Geometry: final body of the model. Coordinates: model frame, mm. Face numbers are marked on the shaded views. A direction names the side the tool comes from. Give positions to 0.01 mm unless a question says otherwise; leave off trailing zeros. Loops run counter-clockwise (first coordinate to the right, second up) from the corner with the lowest first, then second, coordinate; pieces in that order, holes last. Notation, with made-up numbers: M 58,41 L 105,41 A32 cw 105,80 Z; hole C -8.75,-22.5 d8. An arc over 180 degrees is marked long. Put each result on its own line as item: value.
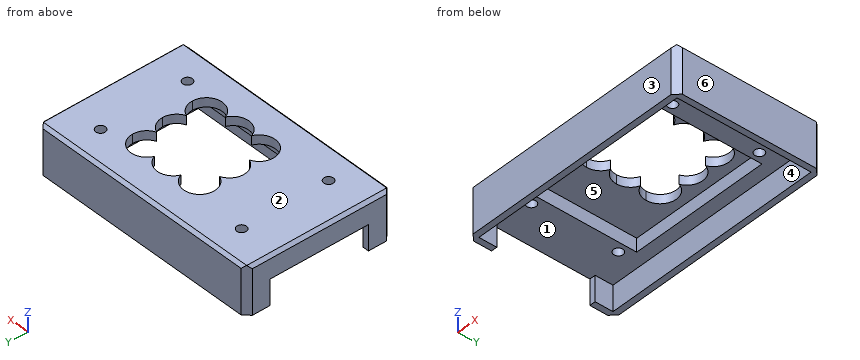
```python
from build123d import *

# Parameters (mm, degrees)
BOSS_EXTRUDE1_START      = 4.485
SKETCH1_W                = 75
SKETCH1_H                = 45
SKETCH1_R                = 1.6
SKETCH1_W_2              = 47.4
SKETCH1_H_2              = 36.3
BOSS_EXTRUDE1_DEPTH      = 3
SKETCH1_4_W              = 75
SKETCH1_4_H              = 45
SKETCH1_4_R              = 1.6
SKETCH1_4_W_2            = 47.4
SKETCH1_4_H_2            = 36.3
BOSS_EXTRUDE2_DEPTH      = 4.485
BOSS_EXTRUDE3_DEPTH      = 8.5
BOSS_EXTRUDE3_DEPTH_BACK = 7.485
SKETCH2_W                = 79
SKETCH2_H                = 49
SKETCH2_W_2              = 75
SKETCH2_H_2              = 45
SKETCH4_W                = 8.5
SKETCH4_H                = 33
CUT_EXTRUDE1_DEPTH       = 52
CHAMFER1_SIZE            = 1
CHAMFER2_SIZE            = 2


with BuildPart() as part:
    # Sketch1 → Boss-Extrude1 (new body)
    # profile 1 of 2: a face of its own
    with BuildSketch(Plane.XY.offset(BOSS_EXTRUDE1_START)):
        with Locations((-52, -40.55)):
            Rectangle(SKETCH1_W, SKETCH1_H)
        with Locations(Location((-78.6, -55.1, 0), (0, 0, 270))):
            Circle(SKETCH1_R, mode=Mode.SUBTRACT)
        with Locations(Location((-78.6, -25.9, 0), (0, 0, 270))):
            Circle(SKETCH1_R, mode=Mode.SUBTRACT)
        with Locations(Location((-25.2, -25.9, 0), (0, 0, 270))):
            Circle(SKETCH1_R, mode=Mode.SUBTRACT)
        with Locations(Location((-25.2, -55.1, 0), (0, 0, 270))):
            Circle(SKETCH1_R, mode=Mode.SUBTRACT)
        with Locations((-51.9, -40.55)):
            Rectangle(SKETCH1_W_2, SKETCH1_H_2, mode=Mode.SUBTRACT)
    # profile 2 of 2: a face of its own
    with BuildSketch(Plane.XY.offset(BOSS_EXTRUDE1_START)):
        with Locations((-51.9, -40.55)):
            Rectangle(SKETCH1_W_2, SKETCH1_H_2)
        with BuildLine():
            ThreePointArc((-35.396713369, -35.7), (-32.895168364, -33.736438417), (-31.95, -30.7))
            ThreePointArc((-31.95, -30.7), (-36.332399876, -25.438227485), (-42.3, -28.796713369))
            ThreePointArc((-42.3, -28.796713369), (-47.3, -25.35), (-52.3, -28.796713369))
            ThreePointArc((-52.3, -28.796713369), (-58.267600124, -25.438227485), (-62.65, -30.7))
            ThreePointArc((-62.65, -30.7), (-61.704831636, -33.736438417), (-59.203286631, -35.7))
            ThreePointArc((-59.203286631, -35.7), (-61.704831636, -37.663561583), (-62.65, -40.7))
            ThreePointArc((-62.65, -40.7), (-61.704831636, -43.736438417), (-59.203286631, -45.7))
            ThreePointArc((-59.203286631, -45.7), (-61.704831636, -47.663561583), (-62.65, -50.7))
            ThreePointArc((-62.65, -50.7), (-58.267600124, -55.961772515), (-52.3, -52.603286631))
            ThreePointArc((-52.3, -52.603286631), (-47.3, -56.05), (-42.3, -52.603286631))
            ThreePointArc((-42.3, -52.603286631), (-36.332399876, -55.961772515), (-31.95, -50.7))
            ThreePointArc((-31.95, -50.7), (-32.895168364, -47.663561583), (-35.396713369, -45.7))
            ThreePointArc((-35.396713369, -45.7), (-32.895168364, -43.736438417), (-31.95, -40.7))
            ThreePointArc((-31.95, -40.7), (-32.895168364, -37.663561583), (-35.396713369, -35.7))
        make_face(mode=Mode.SUBTRACT)
    extrude(amount=BOSS_EXTRUDE1_DEPTH)

    # Sketch1<4> → Boss-Extrude2 (add)
    with BuildSketch(Plane.XY):
        with Locations((-52, -40.55)):
            Rectangle(SKETCH1_4_W, SKETCH1_4_H)
        with Locations((-78.6, -55.1)):
            Circle(SKETCH1_4_R, mode=Mode.SUBTRACT)
        with Locations((-78.6, -25.9)):
            Circle(SKETCH1_4_R, mode=Mode.SUBTRACT)
        with Locations((-25.2, -25.9)):
            Circle(SKETCH1_4_R, mode=Mode.SUBTRACT)
        with Locations((-25.2, -55.1)):
            Circle(SKETCH1_4_R, mode=Mode.SUBTRACT)
        with Locations((-51.9, -40.55)):
            Rectangle(SKETCH1_4_W_2, SKETCH1_4_H_2, mode=Mode.SUBTRACT)
    extrude(amount=BOSS_EXTRUDE2_DEPTH)

    # Sketch2 → Boss-Extrude3 (add, two sides: drawn at the far end of the back side and taken through both)
    with BuildSketch(Plane(origin=(0, 0, 0), x_dir=(-1, 0, 0), z_dir=(0, 0, -1)).offset(-BOSS_EXTRUDE3_DEPTH_BACK)):
        with Locations((52, -40.55)):
            Rectangle(SKETCH2_W, SKETCH2_H)
        with Locations((52, -40.55)):
            Rectangle(SKETCH2_W_2, SKETCH2_H_2, mode=Mode.SUBTRACT)
    extrude(amount=BOSS_EXTRUDE3_DEPTH + BOSS_EXTRUDE3_DEPTH_BACK)

    # Sketch4 → Cut-Extrude1 (cut)
    with BuildSketch(Plane(origin=(-89.5, 0, 0), x_dir=(0, 0, -1), z_dir=(1, 0, 0))):
        with Locations((4.25, -40.55)):
            Rectangle(SKETCH4_W, SKETCH4_H)
    extrude(amount=-CUT_EXTRUDE1_DEPTH, mode=Mode.SUBTRACT)

    # Chamfer1
    chamfer1_edges = [part.edges().sort_by_distance(p)[0] for p in [
        (-52, -65.05, 7.485),
        (-91.5, -40.55, 7.485),
        (-52, -16.05, 7.485),
        (-12.5, -40.55, 7.485),
    ]]
    chamfer(chamfer1_edges, length=CHAMFER1_SIZE)

    # Chamfer2
    chamfer2_edges = [part.edges().sort_by_distance(p)[0] for p in [
        (-12.5, -65.05, -1.0075),
        (-91.5, -65.05, -1.0075),
        (-12.5, -16.05, -1.0075),
        (-91.5, -16.05, -1.0075),
    ]]
    chamfer(chamfer2_edges, length=CHAMFER2_SIZE - 0.0001)  # a hair under: the kernel refuses the full size


solid = part.part
```
Item 1: Pin query (flat end, axial travel): pin 1 Ø4 at (x, y) = (-25.2, -25.9) entering from -Z. Return the tip coordinate at first contact, or that it passes through.
Output values:
pin 1: z = 0
Item 2: Set-up query: the marked faces 5 and 6. Return all of +Z, -Z, +X, -X, +Y, -Y with unobstructed straight access to the full face (end or side cutting, diameter ignored); none if empty.
Output values:
face 5: -Z
face 6: +Z, -Z, +X, +Y, -Y
Item 3: Mould query, pull axis Y, two halves, no side actions, for the marked faces 1, 2, 3 and 4. Classes: pulls with the +Y half, pulls with the -Y half, needs draft (parallel to the pull), parting line crosses it, or undercut.
Output values:
face 1: undercut
face 2: needs draft
face 3: pulls with the -Y half
face 4: undercut
Item 4: Section C-C on x = -33.5. Output: boundary loops of the cut face in (y, z) (3 decimals), then the cut area to 3 significant figures.
Output values:
outline: M -65.05,-8.5 L -63.05,-8.5 L -63.05,0 L -58.7,0 L -58.7,4.485 L -54.466,4.485 L -54.466,7.485 L -64.05,7.485 L -65.05,6.485 Z; M -46.934,4.485 L -44.466,4.485 L -44.466,7.485 L -46.934,7.485 Z; M -36.934,4.485 L -34.466,4.485 L -34.466,7.485 L -36.934,7.485 Z; M -26.934,4.485 L -22.4,4.485 L -22.4,0 L -18.05,0 L -18.05,-8.5 L -16.05,-8.5 L -16.05,6.485 L -17.05,7.485 L -26.934,7.485 Z
area: 169 mm²
Item 5: Section B-B on x = -50.5. Output: boundary loops of the cut face in (y, z) (3 decimals).
Output values:
outline: M -65.05,-8.5 L -63.05,-8.5 L -63.05,0 L -58.7,0 L -58.7,4.485 L -54.987,4.485 L -54.987,7.485 L -64.05,7.485 L -65.05,6.485 Z; M -26.413,4.485 L -22.4,4.485 L -22.4,0 L -18.05,0 L -18.05,-8.5 L -16.05,-8.5 L -16.05,6.485 L -17.05,7.485 L -26.413,7.485 Z
Item 6: Section A-A on z = 2.75. Output: boundary loops of the cut face in (x, y).
Output values:
outline: M -91.5,-63.05 L -89.5,-65.05 L -14.5,-65.05 L -12.5,-63.05 L -12.5,-18.05 L -14.5,-16.05 L -89.5,-16.05 L -91.5,-18.05 Z; hole C -78.6,-55.1 d3.2; hole C -78.6,-25.9 d3.2; hole M -75.6,-58.7 L -28.2,-58.7 L -28.2,-22.4 L -75.6,-22.4 Z; hole C -25.2,-55.1 d3.2; hole C -25.2,-25.9 d3.2
Item 7: Section D-D on x = -83.5. Output: boundary loops of the cut face in (y, z) (3 decimals).
Output values:
outline: M -65.05,-8.5 L -63.05,-8.5 L -63.05,0 L -18.05,0 L -18.05,-8.5 L -16.05,-8.5 L -16.05,6.485 L -17.05,7.485 L -64.05,7.485 L -65.05,6.485 Z
Item 8: Line query: probe 1 along Y at (x, z) = (-78.6, 5.25); probe 2 along X at (y, z) = (-55.1, 2.5); probe 3 along Y at (x, z) = (-65.5, 2.5). Output: solid intervals per line, ascending. Write a range as [from, to].
Output values:
probe 1: [-65.05, -56.7], [-53.5, -27.5], [-24.3, -16.05]
probe 2: [-91.5, -80.2], [-77, -75.6], [-28.2, -26.8], [-23.6, -12.5]
probe 3: [-65.05, -58.7], [-22.4, -16.05]
